Here's how the part is built. I have some questions about the finished solid (model axes, mm). A direction names the side the tool comes from. Give positions to 0.01 mm unless a question says otherwise; leave off trailing zeros. Loops run counter-clockwise (first coordinate to the right, second up) from the corner with the lowest first, then second, coordinate; pieces in that order, holes last.
Q1. If we section it at B-B (x = 0): Please give me the cut outline in (y, z).
Q2. I need wall thicknesses on line 1 (Y direction, x = 0, z = 2.9); line 2 (Y direction, x = 0.5, z = -5.25); line 3 (X direction, y = -29, z = 1.75). Which ranges of each line are inside material? Lowest first, please.
Q3. Will these pins go through, and if not, where does the flat tip stop? P1, Ø4.5, axis at x = 0, y = 10.35, coming from the +Z side; P2, Ø1.1, axis at y = -2, z = -2.5, coming from the -X side; P3, Ø7, axis at x = -27.5, y = -8.5, coming from the +Z side; P4, Ø2, axis at x = 0.5, y = -20, coming from the -Z side.
Q4. For faces 5 (the face through (26, -1, -3.81)), 6 (the face through (-22.727, -1, -2)), 7 (the face through (0, 16.066, -4)), 8 (the face through (0, 48.45, -3)), which set-ups out of +Z, -Z, +X, -X, +Y, -Y let a thin tool reach every point of the face, with its end or its side?
Q5. If we section it at A-A (z = -1.75): Please give me the cut outline in (x, y).
Q6. We'd pull the mould along X, two halves only. Please class faces 1 (the face through (-0.231, -16.843, 1.977)), 2 (the face through (-26, -1, -3.81)), 3 (the face through (-7.83, -1, 2)), 4 (the face through (-2, -17, 0)): +X half, -X half, draft (parallel to the pull), parting line (faces both ways), or undercut.
Q7. If we section it at C-C (y = -33.5): Please give me the cut outline in (x, z).
from build123d import *

# Parameters (mm, degrees)
F1_DEPTH = 48.4505
F2_R     = 1.778
F3_DEPTH = 11.5199
F4_W     = 6.985
F4_H     = 11.43
F4_R     = 1.778
F5_DEPTH = 7.62


with BuildPart() as f1:
    # F0 (on Front) → F1 (new body, symmetric)
    with BuildSketch(Plane.XZ):
        Polygon((-29.07665, -3.81), (-29.07665, -7.62), (29.08935, -7.62), (29.08935, -3.81), (22.73935, -3.81), (22.73935, 0), (7.82955, 0), (7.82955, 3.8989), (-7.82955, 3.8989), (-7.82955, 0), (-22.72665, 0), (-22.72665, -3.81), align=None)
    extrude(amount=F1_DEPTH, both=True)

    # F2 (on face) → F3 (cut, through all)
    with BuildSketch(Plane.XY.offset(3.8989)):
        with Locations((0, 10.3505)):
            Circle(F2_R)
        with Locations((0, -18.6055)):
            Circle(F2_R)
    extrude(amount=-F3_DEPTH, mode=Mode.SUBTRACT)

    # F4 (on face) → F5 (cut, through all)
    with BuildSketch(Plane(origin=(0, 0, -7.62), x_dir=(1, 0, 0), z_dir=(0, 0, -1))):
        with Locations((0, 18.6055)):
            Rectangle(F4_W, F4_H)
        with Locations((0, 18.6055)):
            Circle(F4_R, mode=Mode.SUBTRACT)
        with Locations((0, -10.3505)):
            Rectangle(F4_W, F4_H)
        with Locations((0, -10.3505)):
            Circle(F4_R, mode=Mode.SUBTRACT)
    extrude(amount=-F5_DEPTH, mode=Mode.SUBTRACT)


solid = f1.part
Check sheet entries:
1. outline: (-48.45, -7.62) - (-24.32, -7.62) - (-24.32, 0) - (-20.38, 0) - (-20.38, 3.9) - (-48.45, 3.9) - close; (-16.83, 0) - (-12.89, 0) - (-12.89, -7.62) - (4.64, -7.62) - (4.64, 0) - (8.57, 0) - (8.57, 3.9) - (-16.83, 3.9) - close; (12.13, 0) - (16.07, 0) - (16.07, -7.62) - (48.45, -7.62) - (48.45, 3.9) - (12.13, 3.9) - close
2. line 1: y = -48.45 to -20.38, -16.83 to 8.57, 12.13 to 48.45
2. line 2: y = -48.45 to -24.32, -12.89 to 4.64, 16.07 to 48.45
2. line 3: x = -7.83 to 7.83
3. P1: stops at z = 3.9
3. P2: stops at x = -22.73
3. P3: stops at z = -3.81
3. P4: stops at z = 0
4. face 5: +Z, +X, +Y, -Y
4. face 6: +Z, -X, +Y, -Y
4. face 7: -Z
4. face 8: +Z, -Z, +X, -X, +Y
5. outline: (-22.73, -48.45) - (22.74, -48.45) - (22.74, 48.45) - (-22.73, 48.45) - close; hole (-3.49, -24.32) - (3.49, -24.32) - (3.49, -12.89) - (-3.49, -12.89) - close; hole (-3.49, 4.64) - (3.49, 4.64) - (3.49, 16.07) - (-3.49, 16.07) - close
6. face 1: undercut
6. face 2: draft
6. face 3: -X half
6. face 4: undercut
7. outline: (-29.08, -7.62) - (29.09, -7.62) - (29.09, -3.81) - (22.74, -3.81) - (22.74, 0) - (7.83, 0) - (7.83, 3.9) - (-7.83, 3.9) - (-7.83, 0) - (-22.73, 0) - (-22.73, -3.81) - (-29.08, -3.81) - close
